Verification items for the finished model (mm, model axes). Coordinates: 2 decimals unless noted, no trailing zeros. Write each loop counter-clockwise with the first axis right and the second up, starting at its lowest first coordinate (ties: lowest second). Pieces come first, ordered by that corner, then holes.
```python
from build123d import *

# Parameters (mm, degrees)
F1_DEPTH       = 23.5
F5_R           = 12.75
F6_DEPTH       = 2.5
F8_D           = 5.9
F8_CSINK_D     = 6.8
F8_CSINK_ANGLE = 90
F9_R           = 5.5
F10_DEPTH      = 17.5


# Not quite as in the source:
# - the arcs of a loft's sections are written as splines that run evenly, so that the points pair up as in the source's solid


with BuildPart() as f1:
    # F0 (on Front) → F1 (new body)
    with BuildSketch(Plane.XZ):
        with BuildLine():
            ThreePointArc((0.5997866287, 11.234), (0, 11.85), (-0.5997866287, 11.234))
            ThreePointArc((-0.5997866287, 11.234), (-7.9549512883, 7.9549512883), (-11.234, 0.5997866287))
            ThreePointArc((-11.234, 0.5997866287), (-11.85, 0), (-11.234, -0.5997866287))
            ThreePointArc((-11.234, -0.5997866287), (-7.9549512883, -7.9549512883), (-0.5997866287, -11.234))
            ThreePointArc((-0.5997866287, -11.234), (0, -11.85), (0.5997866287, -11.234))
            ThreePointArc((0.5997866287, -11.234), (7.9549512883, -7.9549512883), (11.234, -0.5997866287))
            ThreePointArc((11.234, -0.5997866287), (11.85, 0), (11.234, 0.5997866287))
            ThreePointArc((11.234, 0.5997866287), (7.9549512883, 7.9549512883), (0.5997866287, 11.234))
        make_face()
    extrude(amount=F1_DEPTH)

    # F1_face (on face) → F4 section 0
    with BuildSketch(Plane.XZ.offset(23.5)):
        with BuildLine():
            add(Edge.make_bspline(
                [(0.5997866287, 11.234), (0.6016799219, 11.3049732474), (0.5908445992, 11.376267359), (0.5450568557, 11.5106795168), (0.5101164815, 11.5737621993), (0.4204642218, 11.6838785828), (0.3657759235, 11.7308833124), (0.2434389451, 11.8029722112), (0.1758224517, 11.8280374139), (0.0360563953, 11.853109213), (-0.0360563953, 11.853109213), (-0.1758224517, 11.8280374139), (-0.2434389451, 11.8029722112), (-0.3657759235, 11.7308833124), (-0.4204642218, 11.6838785828), (-0.5101164815, 11.5737621993), (-0.5450568557, 11.5106795168), (-0.5908445992, 11.376267359), (-0.6016799219, 11.3049732474), (-0.5997866287, 11.234)],
                knots=[0, 0, 0, 0, 0.1111111111, 0.1111111111, 0.2222222222, 0.2222222222, 0.3333333333, 0.3333333333, 0.4444444444, 0.4444444444, 0.5555555556, 0.5555555556, 0.6666666667, 0.6666666667, 0.7777777778, 0.7777777778, 0.8888888889, 0.8888888889, 1, 1, 1, 1], degree=3))
            add(Edge.make_bspline(
                [(-0.5997866287, 11.234), (-1.9704441734, 11.1608201827), (-3.3271537618, 10.8340484232), (-5.834489174, 9.7162386482), (-6.984369661, 8.9255329157), (-8.9255329157, 6.984369661), (-9.7162386482, 5.834489174), (-10.8340484232, 3.3271537618), (-11.1608201827, 1.9704441734), (-11.234, 0.5997866287)],
                knots=[0, 0, 0, 0, 0.25, 0.25, 0.5, 0.5, 0.75, 0.75, 1, 1, 1, 1], degree=3))
            add(Edge.make_bspline(
                [(-11.234, 0.5997866287), (-11.3049732474, 0.6016799219), (-11.376267359, 0.5908445992), (-11.5106795168, 0.5450568557), (-11.5737621993, 0.5101164815), (-11.6838785828, 0.4204642218), (-11.7308833124, 0.3657759235), (-11.8029722112, 0.2434389451), (-11.8280374139, 0.1758224517), (-11.853109213, 0.0360563953), (-11.853109213, -0.0360563953), (-11.8280374139, -0.1758224517), (-11.8029722112, -0.2434389451), (-11.7308833124, -0.3657759235), (-11.6838785828, -0.4204642218), (-11.5737621993, -0.5101164815), (-11.5106795168, -0.5450568557), (-11.376267359, -0.5908445992), (-11.3049732474, -0.6016799219), (-11.234, -0.5997866287)],
                knots=[0, 0, 0, 0, 0.1111111111, 0.1111111111, 0.2222222222, 0.2222222222, 0.3333333333, 0.3333333333, 0.4444444444, 0.4444444444, 0.5555555556, 0.5555555556, 0.6666666667, 0.6666666667, 0.7777777778, 0.7777777778, 0.8888888889, 0.8888888889, 1, 1, 1, 1], degree=3))
            add(Edge.make_bspline(
                [(-11.234, -0.5997866287), (-11.1608201827, -1.9704441734), (-10.8340484232, -3.3271537618), (-9.7162386482, -5.834489174), (-8.9255329157, -6.984369661), (-6.984369661, -8.9255329157), (-5.834489174, -9.7162386482), (-3.3271537618, -10.8340484232), (-1.9704441734, -11.1608201827), (-0.5997866287, -11.234)],
                knots=[0, 0, 0, 0, 0.25, 0.25, 0.5, 0.5, 0.75, 0.75, 1, 1, 1, 1], degree=3))
            add(Edge.make_bspline(
                [(-0.5997866287, -11.234), (-0.6016799219, -11.3049732474), (-0.5908445992, -11.376267359), (-0.5450568557, -11.5106795168), (-0.5101164815, -11.5737621993), (-0.4204642218, -11.6838785828), (-0.3657759235, -11.7308833124), (-0.2434389451, -11.8029722112), (-0.1758224517, -11.8280374139), (-0.0360563953, -11.853109213), (0.0360563953, -11.853109213), (0.1758224517, -11.8280374139), (0.2434389451, -11.8029722112), (0.3657759235, -11.7308833124), (0.4204642218, -11.6838785828), (0.5101164815, -11.5737621993), (0.5450568557, -11.5106795168), (0.5908445992, -11.376267359), (0.6016799219, -11.3049732474), (0.5997866287, -11.234)],
                knots=[0, 0, 0, 0, 0.1111111111, 0.1111111111, 0.2222222222, 0.2222222222, 0.3333333333, 0.3333333333, 0.4444444444, 0.4444444444, 0.5555555556, 0.5555555556, 0.6666666667, 0.6666666667, 0.7777777778, 0.7777777778, 0.8888888889, 0.8888888889, 1, 1, 1, 1], degree=3))
            add(Edge.make_bspline(
                [(0.5997866287, -11.234), (1.9704441734, -11.1608201827), (3.3271537618, -10.8340484232), (5.834489174, -9.7162386482), (6.984369661, -8.9255329157), (8.9255329157, -6.984369661), (9.7162386482, -5.834489174), (10.8340484232, -3.3271537618), (11.1608201827, -1.9704441734), (11.234, -0.5997866287)],
                knots=[0, 0, 0, 0, 0.25, 0.25, 0.5, 0.5, 0.75, 0.75, 1, 1, 1, 1], degree=3))
            add(Edge.make_bspline(
                [(11.234, -0.5997866287), (11.3049732474, -0.6016799219), (11.376267359, -0.5908445992), (11.5106795168, -0.5450568557), (11.5737621993, -0.5101164815), (11.6838785828, -0.4204642218), (11.7308833124, -0.3657759235), (11.8029722112, -0.2434389451), (11.8280374139, -0.1758224517), (11.853109213, -0.0360563953), (11.853109213, 0.0360563953), (11.8280374139, 0.1758224517), (11.8029722112, 0.2434389451), (11.7308833124, 0.3657759235), (11.6838785828, 0.4204642218), (11.5737621993, 0.5101164815), (11.5106795168, 0.5450568557), (11.376267359, 0.5908445992), (11.3049732474, 0.6016799219), (11.234, 0.5997866287)],
                knots=[0, 0, 0, 0, 0.1111111111, 0.1111111111, 0.2222222222, 0.2222222222, 0.3333333333, 0.3333333333, 0.4444444444, 0.4444444444, 0.5555555556, 0.5555555556, 0.6666666667, 0.6666666667, 0.7777777778, 0.7777777778, 0.8888888889, 0.8888888889, 1, 1, 1, 1], degree=3))
            add(Edge.make_bspline(
                [(11.234, 0.5997866287), (11.1608201827, 1.9704441734), (10.8340484232, 3.3271537618), (9.7162386482, 5.834489174), (8.9255329157, 6.984369661), (6.984369661, 8.9255329157), (5.834489174, 9.7162386482), (3.3271537618, 10.8340484232), (1.9704441734, 11.1608201827), (0.5997866287, 11.234)],
                knots=[0, 0, 0, 0, 0.25, 0.25, 0.5, 0.5, 0.75, 0.75, 1, 1, 1, 1], degree=3))
        make_face()
    # F3 (on offset) → F4 section 1
    with BuildSketch(Plane.XZ.offset(25)):
        with BuildLine():
            add(Edge.make_bspline(
                [(-0.5464722617, 10.2354222222), (-1.8862858976, 10.1638891704), (-3.2113491637, 9.8259836202), (-5.6322529271, 8.6683588136), (-6.7271409022, 7.8490950331), (-7.6239507036, 6.8511222196)],
                knots=[0, 0, 0, 0, 0.5, 0.5, 1, 1, 1, 1], degree=3))
            add(Edge.make_bspline(
                [(-7.6239507036, 6.8511222196), (-8.5207605051, 5.8531494062), (-9.2187864201, 4.6772528793), (-10.112059537, 2.1468510607), (-10.306955274, 0.7933413741), (-10.2354222222, -0.5464722617)],
                knots=[0, 0, 0, 0, 0.5, 0.5, 1, 1, 1, 1], degree=3))
            add(Edge.make_bspline(
                [(-10.2354222222, -0.5464722617), (-10.1638891704, -1.8862858976), (-9.8259836202, -3.2113491637), (-8.6683588136, -5.6322529271), (-7.8490950331, -6.7271409022), (-6.8511222196, -7.6239507036)],
                knots=[0, 0, 0, 0, 0.5, 0.5, 1, 1, 1, 1], degree=3))
            add(Edge.make_bspline(
                [(-6.8511222196, -7.6239507036), (-5.8531494062, -8.5207605051), (-4.6772528793, -9.2187864201), (-2.1468510607, -10.112059537), (-0.7933413741, -10.306955274), (0.5464722617, -10.2354222222)],
                knots=[0, 0, 0, 0, 0.5, 0.5, 1, 1, 1, 1], degree=3))
            add(Edge.make_bspline(
                [(0.5464722617, -10.2354222222), (1.8862858976, -10.1638891704), (3.2113491637, -9.8259836202), (5.6322529271, -8.6683588136), (6.7271409022, -7.8490950331), (7.6239507036, -6.8511222196)],
                knots=[0, 0, 0, 0, 0.5, 0.5, 1, 1, 1, 1], degree=3))
            add(Edge.make_bspline(
                [(7.6239507036, -6.8511222196), (8.5207605051, -5.8531494062), (9.2187864201, -4.6772528793), (10.112059537, -2.1468510607), (10.306955274, -0.7933413741), (10.2354222222, 0.5464722617)],
                knots=[0, 0, 0, 0, 0.5, 0.5, 1, 1, 1, 1], degree=3))
            add(Edge.make_bspline(
                [(10.2354222222, 0.5464722617), (10.1638891704, 1.8862858976), (9.8259836202, 3.2113491637), (8.6683588136, 5.6322529271), (7.8490950331, 6.7271409022), (6.8511222196, 7.6239507036)],
                knots=[0, 0, 0, 0, 0.5, 0.5, 1, 1, 1, 1], degree=3))
            add(Edge.make_bspline(
                [(6.8511222196, 7.6239507036), (5.8531494062, 8.5207605051), (4.6772528793, 9.2187864201), (2.1468510607, 10.112059537), (0.7933413741, 10.306955274), (-0.5464722617, 10.2354222222)],
                knots=[0, 0, 0, 0, 0.5, 0.5, 1, 1, 1, 1], degree=3))
        make_face()
    loft(ruled=True)

    # F5 (on face) → F6 (join)
    with BuildSketch(Plane(origin=(0, 0, 0), x_dir=(-1, 0, 0), z_dir=(0, 1, 0))):
        Circle(F5_R)
    extrude(amount=F6_DEPTH)

    # F8 (through all)
    with Locations(Plane(origin=(0, 2.5, 0), x_dir=(-1, 0, 0), z_dir=(0, 1, 0))):
        with Locations((0, 0)):
            CounterSinkHole(F8_D / 2, F8_CSINK_D / 2, counter_sink_angle=F8_CSINK_ANGLE)

    # F9 (on face) → F10 (cut)
    with BuildSketch(Plane.XZ.offset(25)):
        Circle(F9_R)
    extrude(amount=-F10_DEPTH, mode=Mode.SUBTRACT)


solid = f1.part
```
1. Sectioned sample at B-B, the plane y = -5. Record the boundary of the cut face in (x, z).
2. Material ranges on L1, parallel to X at y = -0.25, z = 0; L2, parallel to Z at x = 0, y = -16, recorded low to high.
3. Sectioned sample at A-A, the plane y = -8.75. Record the boundary of the cut face in (x, z).
4. Gauge pin test, flat ends, axial feed: P1, Ø3, axis at x = 5, y = -8, coming from the -Z side; P2, Ø4, axis at x = 2, y = -18, coming from the -Z side; P3, Ø1, axis at x = -5.5, y = -22, coming from the -Z side. Record the tip position at first contact, or that the pin passes through.
5. Draft check along Y on faces 1 (the flat face through (2.4, -7.5, -2.4)), 2 (the cylindrical face through (11.85, -11.59, -0.01)), 3 (the cylindrical face through (-1.19, -16.37, -5.37)). Enter one of: pulls with the +Y half, pulls with the -Y half, needs draft (parallel to the pull), parting line crosses it, or undercut.
Outcome:
1. outline: (-11.23, -0.6) arc R11.25 ccw to (-0.6, -11.23) arc R0.6 ccw (long way) to (0.6, -11.23) arc R11.25 ccw to (11.23, -0.6) arc R0.6 ccw (long way) to (11.23, 0.6) arc R11.25 ccw to (0.6, 11.23) arc R0.6 ccw (long way) to (-0.6, 11.23) arc R11.25 ccw to (-11.23, 0.6) arc R0.6 ccw (long way) to start; hole circle Ø5.9 at (0, 0)
2. L1: x = -11.85 to -2.95, 2.95 to 11.85
2. L2: z = -11.85 to -5.5, 5.5 to 11.85
3. outline: (-11.23, -0.6) arc R11.25 ccw to (-0.6, -11.23) arc R0.6 ccw (long way) to (0.6, -11.23) arc R11.25 ccw to (11.23, -0.6) arc R0.6 ccw (long way) to (11.23, 0.6) arc R11.25 ccw to (0.6, 11.23) arc R0.6 ccw (long way) to (-0.6, 11.23) arc R11.25 ccw to (-11.23, 0.6) arc R0.6 ccw (long way) to start; hole circle Ø11 at (0, 0)
4. P1: stops at z = -10.69
4. P2: stops at z = -11.85
4. P3: stops at z = -10.08
5. face 1: pulls with the -Y half
5. face 2: undercut
5. face 3: needs draft
